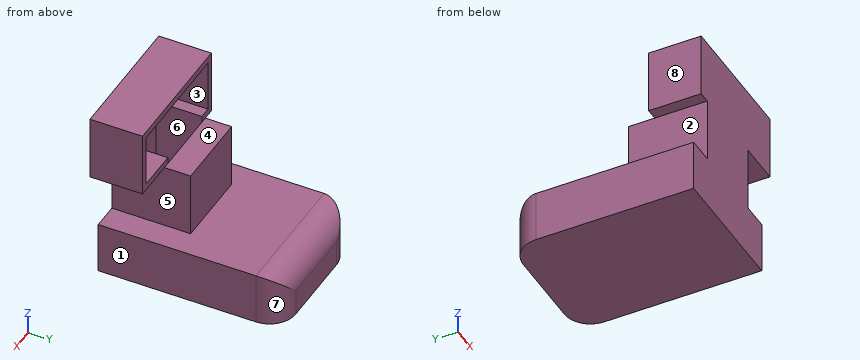
from build123d import *

# Parameters (mm, degrees)
F0_W        = 70
F0_H        = 20
F1_DEPTH    = 25
F2_W        = 30
F2_H        = 30
F3_DEPTH    = 25
F4_R        = 10
F5_W        = 50.5173448473
F5_H        = 20
F6_DEPTH    = 25
F7_T        = 2.5
F7_T3_DEPTH = 35
F7_T5_DEPTH = 35
F7_T7_DEPTH = 25


# Not quite as in the source:
# - a shell that OpenCascade refuses in one call is made with other operations: the cavity is built on its own and cut out


with BuildPart() as f1:
    # F0 (on Right) → F1 (new body, symmetric)
    with BuildSketch(Plane.YZ):
        with Locations((35, 10)):
            Rectangle(F0_W, F0_H)
    extrude(amount=F1_DEPTH, both=True)

    # F2 (on face) → F3 (join)
    with BuildSketch(Plane.XY.offset(20)):
        with Locations((0, 15)):
            Rectangle(F2_W, F2_H)
    extrude(amount=F3_DEPTH)

    # F4
    f4_edges = [f1.edges().sort_by_distance(p)[0] for p in [
        (-25, 70, 10),
        (0, 70, 20),
        (25, 70, 10),
    ]]
    fillet(f4_edges, radius=F4_R)

    # F5 (on face) → F6 (join)
    with BuildSketch(Plane.XY.offset(45)):
        with Locations((5.7856766507, 10)):
            Rectangle(F5_W, F5_H)
    extrude(amount=F6_DEPTH)

    # F7: shell of thickness 2.5, made by hand


with BuildPart() as f7_core1:
    # F7_t2: copy of F1
    add(f1.part)

    # the walls: a layer under each face that stays
    f7_faces = [f7_core1.faces().sort_by_distance(p)[0] for p in [
        (-16.6666666667, 50, 20),
        (25, 30, 10),
        (0, 67.0710678119, 17.0710678119),
        (3.0221745372, 0, 35),
        (-25, 30, 10),
        (15, 15, 32.5),
        (0, 30, 32.5),
        (-15, 15, 32.5),
        (22.0710678119, 67.0710678119, 10),
        (0, 35, 0),
        (0, 70, 5),
        (-22.0710678119, 67.0710678119, 10),
        (23.0221745372, 10, 45),
        (0, 25, 45),
        (-17.2364978865, 10, 45),
        (-19.472995773, 10, 57.5),
        (31.0443490744, 10, 57.5),
        (5.7856766507, 10, 70),
    ]]
    thicken(f7_faces, amount=-F7_T, mode=Mode.SUBTRACT)

    # F7_s4 → F7_t3 (cut)
    with BuildSketch(Plane.XZ.offset(-32.5)):
        Polygon((15.025, 20.025), (15, 17.5), (12.5, 17.5), (12.5, 20), align=None)
        Polygon((-15.025, 20.025), (-15, 17.5), (-12.5, 17.5), (-12.5, 20), align=None)
    extrude(amount=F7_T3_DEPTH, mode=Mode.SUBTRACT)

    # F7_s6 → F7_t5 (cut)
    with BuildSketch(Plane.YZ.offset(-17.5)):
        Polygon((30.025, 20.025), (30, 17.5), (27.5, 17.5), (27.5, 20), align=None)
    extrude(amount=F7_T5_DEPTH, mode=Mode.SUBTRACT)

    # F7_s8 → F7_t7 (cut)
    with BuildSketch(Plane.XZ.offset(-22.5)):
        Polygon((15.025, 44.975), (12.5, 45), (12.5, 47.5), (15, 47.5), align=None)
        Polygon((-15.025, 44.975), (-12.5, 45), (-12.5, 47.5), (-15, 47.5), align=None)
    extrude(amount=F7_T7_DEPTH, mode=Mode.SUBTRACT)


with BuildPart() as f1_1:
    add(f1.part)

    # what is left inside the walls is the cavity
    f7_cavity = [f7_core1.part.solids().sort_by_distance(p)[0] for p in [
        (-7.5, 35, 2.525),
    ]]
    add(f7_cavity, mode=Mode.SUBTRACT)


solid = f1_1.part
Geometry: final body of the model. Coordinates: model frame, mm. Face numbers are marked on the shaded views. A direction names the side the tool comes from. Give positions to 0.01 mm unless a question says otherwise; leave off trailing zeros. Loops run counter-clockwise (first coordinate to the right, second up) from the corner with the lowest first, then second, coordinate; pieces in that order, holes last. Notation, with made-up numbers: (9, 29) - (49, 29) arc R27 cw to (49, 67) - close; hole circle Ø5 at (74.5, 42). An arc over 180 degrees is marked (long way). One line per question, with ' | ' between items. Start each with the question number.
(1) Section query D-D on x = -8.5. Return loops of the section in (y, z), then the cut area to 3 significant figures.
(2) Section query A-A on z = 30. Return loops of the section in (x, y).
(3) Section query B-B on x = 20.5. Return loops of the section in (y, z), then the cut area to 3 significant figures.
(4) Ray query, line 1 (X direction, y = 5, z = 13); line 2 (X direction, y = 5.5, z = 58); line 3 (Z direction, x = 26.5, y = 7.5). Return the intervals inside material, ascending. Write a range as from..to.
(5) Section query C-C on y = 5. Return loops of the section in (x, z), then the cut area to 3 significant figures.
(6) Contact query for flat-ended pins moving along their axis: pin 1 (4 mm diameter, centred on y = 18.5, z = 31.5, fed in from -X); pin 2 (3 mm diameter, centred on y = 61, z = 16, fed in from +X); pin 3 (12.5 mm diameter, centred on x = 4.5, z = 27.5, fed in from +Y). Output: stop coordinate, or through.
(7) Reachability of the marked faces 1, 2, 3, 4 and 5 from +Z, -Z, +X, -X, +Y, -Y: full face, straight path, thin tool, end or side. Return the list, or none.
(8) Pull-direction query (X, two-part tool) for the marked faces 6, 7 and 8; classes: released by +X, released by -X, zero draft, split by the parting line, or undercut.
The answers:
1) outline: (0, 0) - (70, 0) - (70, 10) arc R10 ccw to (60, 20) - (30, 20) - (30, 45) - (20, 45) - (20, 42.5) - (27.5, 42.5) - (27.5, 17.5) - (60, 17.5) arc R7.5 cw to (67.5, 10) - (67.5, 2.5) - (2.5, 2.5) - (2.5, 67.5) - (20, 67.5) - (20, 70) - (0, 70) - close | area: 603 mm2
2) outline: (-15, 0) - (15, 0) - (15, 30) - (-15, 30) - close; hole (-12.5, 2.5) - (12.5, 2.5) - (12.5, 27.5) - (-12.5, 27.5) - close
3) outline: (0, 0) - (68.35, 0) - (68.35, 15.5) arc R10 ccw to (60, 20) - (0, 20) - close; (0, 45) - (20, 45) - (20, 47.5) - (2.5, 47.5) - (2.5, 67.5) - (20, 67.5) - (20, 70) - (0, 70) - close; hole (2.5, 2.5) - (65.1, 2.5) - (65.1, 15.5) arc R7.5 ccw to (60, 17.5) - (2.5, 17.5) - close | area: 570 mm2
4) line 1: -25..-22.5, 22.5..25 | line 2: -19.47..-16.97, 28.54..31.04 | line 3: 45..47.5, 67.5..70
5) outline: (-25, 0) - (25, 0) - (25, 20) - (15, 20) - (15, 45) - (31.04, 45) - (31.04, 70) - (-19.47, 70) - (-19.47, 45) - (-15, 45) - (-15, 20) - (-25, 20) - close; hole (-22.5, 2.5) - (22.5, 2.5) - (22.5, 17.5) - (12.5, 17.5) - (12.5, 47.5) - (28.54, 47.5) - (28.54, 67.5) - (-16.97, 67.5) - (-16.97, 47.5) - (-12.5, 47.5) - (-12.5, 17.5) - (-22.5, 17.5) - close | area: 678 mm2
6) pin 1: x = -15 | pin 2: x = 25 | pin 3: y = 30
7) face 1: -Z, +X, +Y, -Y | face 2: -X, +Y, -Y | face 3: +Y | face 4: +Z, +X, -X, +Y | face 5: +X, +Y, -Y
8) face 6: undercut | face 7: released by +X | face 8: released by -X
